Read the model definition and answer for the solid it produces. Units are mm, in the model's axes. A direction names the side the tool comes from. Give positions to 0.01 mm unless a question says otherwise; leave off trailing zeros. Loops run counter-clockwise (first coordinate to the right, second up) from the corner with the lowest first, then second, coordinate; pieces in that order, holes last. Notation, with made-up numbers: (51.25, 0.25) -> (63.25, 0.25) arc R16 cw to (63.25, 13.25) -> close; hole circle Ø8 at (69, 79.5). An arc over 180 degrees is marked (long way). Return JSON: item names as keys, results as strings. Group by question number.
Autodesk Inventor part; units mm, degrees
ref_plane "YZ Plane" through (0, 0, 0) normal (1, 0, 0) x (0, 1, 0)
ref_plane "XZ Plane" through (0, 0, 0) normal (0, 1, 0) x (-1, 0, 0)
ref_plane "XY Plane" through (0, 0, 0) normal (0, 0, 1) x (1, 0, 0)
sketch "Sketch1" plane through (0, 0, 0) normal (0, 0, 1) x (1, 0, 0)
  circle A0 centre (0, 0) radius 6
  circle A1 centre (-1.5, 0) radius 1.6
  dimension "d1" = 12
  dimension "d8" = 3.2
  dimension "d9" = 1.5
extrude "Extrusion1" add sketch "Sketch1" along normal blind 20
sketch "Sketch2" plane through (0, 0, 20) normal (0, 0, 1) x (1, 0, 0)
  circle A0 centre (0, 0) radius 3.9
  circle A1 centre (-1.5, 0) radius 1.6
  dimension "d4" = 7.8
extrude "Extrusion2" add sketch "Sketch2" along normal blind 3
sketch "Sketch3" plane through (0, 0, 0) normal (0, 0, -1) x (-1, 0, 0)
  circle A0 centre (0, 0) radius 8
  circle A1 centre (0, 0) radius 6
  dimension "d10" = 16
extrude "Extrusion3" add sketch "Sketch3" against normal blind 2
sketch "Sketch5" plane through (0, 0, 0) normal (1, 0, 0) x (0, 1, 0)
  line L0 (-44, 2) -> (-4, 2)
  line L1 (-4, 2) -> (-4, 12)
  line L2 (-4, 12) -> (-44, 12)
  line L3 (-44, 12) -> (-44, 2)
  line L4 (-8, 0) -> (8, 0)
  line L5 (-8, 0) -> (-8, 2)
  point P0 (0, 0)
  dimension "d22" = 40
  dimension "d24" = 10
  dimension "d25" = 4
  dimension "d26" = 0
extrude "Extrusion5" add sketch "Sketch5" along normal mid plane 4
properties part number "spacer off center"
1. Which of the six approach directions +Z, -Z, +X, -X, +Y, -Y give full straight-line access (tool end or side, diameter ignored) to faces 1 (the flat face through (0, -44, 7)), 2 (the flat face through (0, -25, 12)), 3 (the cylindrical face through (-2.87, -2.64, 21.48))?
2. Determine the mould class of faces 4 (the cylindrical face through (0.026, -0.481, 11.339)), 5 (the flat face through (2, -25, 7)), 6 (the flat face through (0, -26, 2)), 7 (the cylindrical face through (-1.301, 5.857, 10.874)) for opening direction X: pulls with the +X half, pulls with the -X half, needs draft (parallel to the pull), parting line crosses it, or undercut.
3. Section A-A on y = 0 is taken. Determine the outline of the cut face in (x, z), then the cut area to 3 significant figures.
4. Section D-D on x = -5.5 is taken. Determine the outline of the cut face in (y, z).
5. Straight lines are drawn through the part: line 1 (Z direction, x = 3, y = -7); line 2 (Y direction, x = -1.5, z = 12.25); line 3 (Y direction, x = -1.5, z = 9.75). For each, find the intervals that lie inside material, in ascending order. Write a range as from..to.
6. Section B-B on x = -1.5 is taken. Determine the outline of the cut face in (y, z), then the cut area to 3 significant figures.
7. Flat-ended cylindrical pins translate along their axes: pin 1 Ø5 at (y, z) = (-30, 5) entering from -X; pin 2 Ø4 at (y, z) = (-29.5, 7.5) entering from +X; pin 3 Ø8 at (x, y) = (-3, -36.5) entering from -Z. Find the tip coordinate at first contact, or state that the pin passes through.
8. Section C-C on z = 12.5 is taken. Determine the outline of the cut face in (x, y).
Completed:
{
 "1": {"face 1": "+Z, -Z, +X, -X, -Y", "face 2": "+Z, +X, -X, -Y", "face 3": "+Z"},
 "2": {"face 4": "undercut", "face 5": "pulls with the +X half", "face 6": "needs draft", "face 7": "parting line crosses it"},
 "3": {"outline": "(-8, 0) -> (-3.1, 0) -> (-3.1, 23) -> (-3.9, 23) -> (-3.9, 20) -> (-6, 20) -> (-6, 2) -> (-8, 2) -> close; (0.1, 0) -> (8, 0) -> (8, 2) -> (6, 2) -> (6, 20) -> (3.9, 20) -> (3.9, 23) -> (0.1, 23) -> close", "area": "198 mm²"},
 "4": {"outline": "(-5.81, 0) -> (5.81, 0) -> (5.81, 2) -> (2.4, 2) -> (2.4, 20) -> (-2.4, 20) -> (-2.4, 2) -> (-5.81, 2) -> close"},
 "5": {"line 1": "z = 0..2", "line 2": "y = -5.81..-1.6, 1.6..5.81", "line 3": "y = -44..-1.6, 1.6..5.81"},
 "6": {"outline": "(-44, 2) -> (-7.86, 2) -> (-7.86, 0) -> (-1.6, 0) -> (-1.6, 23) -> (-3.6, 23) -> (-3.6, 20) -> (-5.81, 20) -> (-5.81, 12) -> (-44, 12) -> close; (1.6, 0) -> (7.86, 0) -> (7.86, 2) -> (5.81, 2) -> (5.81, 20) -> (3.6, 20) -> (3.6, 23) -> (1.6, 23) -> close", "area": "570 mm²"},
 "7": {"pin 1": "stops at x = -2", "pin 2": "stops at x = 2", "pin 3": "stops at z = 2"},
 "8": {"outline": "circle Ø12 at (0, 0); hole circle Ø3.2 at (-1.5, 0)"}
}
